from build123d import *

# Parameters (mm, degrees)
SKETCH1_R           = 13
BOSS_EXTRUDE1_DEPTH = 6
SKETCH2_W           = 20
SKETCH2_H           = 10
SKETCH2_R           = 3
BOSS_EXTRUDE2_DEPTH = 6


with BuildPart() as part:
    # Sketch1 → Boss-Extrude1 (new body)
    with BuildSketch(Plane.XY):
        with BuildLine():
            Line((-25, -120), (25, -120))
            Line((25, -120), (25, 120))
            ThreePointArc((25, 120), (0, 145), (-25, 120))
            Line((-25, 120), (-25, -120))
        make_face()
        with Locations((0, 120)):
            Circle(SKETCH1_R, mode=Mode.SUBTRACT)
    extrude(amount=BOSS_EXTRUDE1_DEPTH)

    # Sketch2 → Boss-Extrude2 (add)
    with BuildSketch(Plane(origin=(0, 0, 0), x_dir=(-1, 0, 0), z_dir=(0, 0, -1))):
        with Locations((0, -125)):
            Rectangle(SKETCH2_W, SKETCH2_H)
        with Locations((0, -125)):
            Circle(SKETCH2_R, mode=Mode.SUBTRACT)
    extrude(amount=-BOSS_EXTRUDE2_DEPTH)


solid = part.part
Verification items for the finished model (mm, model axes). A direction names the side the tool comes from. Coordinates: 2 decimals unless noted, no trailing zeros. Write each loop counter-clockwise with the first axis right and the second up, starting at its lowest first coordinate (ties: lowest second). Pieces come first, ordered by that corner, then holes. Notation, with made-up numbers: M -1,-36.75 L 29,-36.75 A19 cw 29,-6.75 Z; hole C 71,-1.5 d6. An arc over 180 degrees is marked long. Use a Markdown table: item, result.
Q1. Go/stop test with flat-tipped pins: P1, Ø3, axis at y = -125, z = 2.5, coming from the +X side; P2, Ø3, axis at y = -127, z = 4, coming from the -X side; P3, Ø3, axis at x = -16.5, z = 1, coming from the -Y side. Record where each tip stops, or that it passes through.
Reply:
| item | result |
|---|---|
| P1 | stops at x = 10 |
| P2 | stops at x = -10 |
| P3 | stops at y = -120 |
Q2. Draft check along Y on faces 4 (the face through (0, -122, 3)), 5 (the face through (0.55, 144.994, 2.958)), 6 (the face through (25, -2, 3)), 7 (the face through (17, -120, 3)). Enter one of: +Y half, -Y half, draft (parallel to the pull), parting line (faces both ways), or undercut.
Reply:
| item | result |
|---|---|
| face 4 | undercut |
| face 5 | +Y half |
| face 6 | draft |
| face 7 | -Y half |
Q3. Sectioned sample at D-D, the plane x = 15.5. Record the boundary of the cut face in (y, z).
Reply:
| item | result |
|---|---|
| outline | M -120,0 L 139.62,0 L 139.62,6 L -120,6 Z |
Q4. Sectioned sample at C-C, the plane x = -6. Record the boundary of the cut face in (y, z), plus the area to 3 significant figures.
Reply:
| item | result |
|---|---|
| outline | M -130,0 L 108.47,0 L 108.47,6 L -130,6 Z; M 131.53,0 L 144.27,0 L 144.27,6 L 131.53,6 Z |
| area | 1,510 mm² |
Q5. Sectioned sample at A-A, the plane z = 3.6. Record the boundary of the cut face in (x, y).
Reply:
| item | result |
|---|---|
| outline | M -25,-120 L -10,-120 L -10,-130 L 10,-130 L 10,-120 L 25,-120 L 25,120 A25 ccw -25,120 Z; hole C 0,120 d26; hole C 0,-125 d6 |
Q6. Set-up check for faces 1 (the face through (-10, -125, 3)), 2 (the face through (-25, 2, 3)), 3 (the face through (10, -125, 3)): record each of +Z, -Z, +X, -X, +Y, -Y from which the full face is reachable in a straight line by a thin tool's end or side.
Reply:
| item | result |
|---|---|
| face 1 | +Z, -Z, -X, -Y |
| face 2 | +Z, -Z, -X, +Y, -Y |
| face 3 | +Z, -Z, +X, -Y |
Q7. Sectioned sample at B-B, the plane y = -125. Record the boundary of the cut face in (x, z).
Reply:
| item | result |
|---|---|
| outline | M -10,0 L -3,0 L -3,6 L -10,6 Z; M 3,0 L 10,0 L 10,6 L 3,6 Z |
Q8. Thickness scan on line 1 (Y direction, x = 0, z = 1.7); line 2 (Y direction, x = 19.5, z = 5.35); line 3 (Y direction, x = 13.5, z = 1.5). Record the ranges inside material, lowest first.
Reply:
| item | result |
|---|---|
| line 1 | y = -130 to -128, -122 to 107, 133 to 145 |
| line 2 | y = -120 to 135.64 |
| line 3 | y = -120 to 141.04 |
